For this review, take the finished solid that the model builds, in its own axes (mm). A direction names the side the tool comes from. Coordinates: 2 decimals unless noted, no trailing zeros. Loops run counter-clockwise (first coordinate to the right, second up) from the corner with the lowest first, then second, coordinate; pieces in that order, holes last. Notation, with made-up numbers: (-29.75, 4) - (5.25, 4) arc R21 ccw to (5.25, 33) - close; hole circle Ø6 at (5, -6). An arc over 180 degrees is marked (long way). One line per item, written item: value. Start each with the question number.
1. To check wall thickness, follow line 1 (X direction, y = 3.5, z = 0); line 2 (X direction, y = 0.75, z = 0); line 3 (X direction, y = 3, z = 6). State the ranges of each line that lie inside material, in increasing order. Write a range as from..to.
2. For faces 1 (the face through (8, 5.4, -8)), 2 (the face through (4.1, 4.4, 0)), 3 (the face through (7, 1.1, 5)), list the 3-axis set-ups (+Z, -Z, +X, -X, +Y, -Y) from which the entire face can be reached by the end or side of a thin tool; tool diameter is ignored.
3. Take a section at A-A, the plane x = 0. State the section outline as (y, z) points.
4. The part is to be moulded in two halves that separate along Z. For faces 4 (the face through (-5.9, 3, 10)), 5 (the face through (0, -1, 6)), 6 (the face through (-6.19, 3.28, 7.484)), 7 (the face through (-1, 3.9, -10)), say which applies: released by +Z, released by -Z, zero draft, split by the parting line, or undercut.
5. Take a section at D-D, the plane x = -8.5. State the section outline as (y, z) points, and give its area (3 significant figures).
6. Take a section at C-C, the plane y = 1.5. Count the separate pieces of the cut face and the enclosed holes in it, and give its area (3 significant figures).
7. Take a section at B-B, the plane z = 0. State the section outline as (x, y) points, and give its area (3 significant figures).
8. Insertion check: pin 1 (4 mm diameter, centred on y = 4, z = -4.5, fed in from +X); pin 2 (12 mm diameter, centred on x = 9, z = 9.5, fed in from -Y); pin 3 (2.5 mm diameter, centred on x = -2, y = 3, fed in from +Z). Each pin has a flat end and moves straight along its axis. Give the tip position at first contact, or say it passes through.
```python
from build123d import *

# Parameters (mm, degrees)
SKETCH1_R           = 12
BOSS_EXTRUDE1_DEPTH = 5.4
CUT_EXTRUDE1_START  = -4.2
CUT_EXTRUDE1_DEPTH  = 4.2
BOSS_EXTRUDE2_DEPTH = 1
SKETCH4_R           = 2.5
SKETCH4_R_2         = 2
CUT_EXTRUDE2_DEPTH  = 11
SKETCH5_R           = 2
BOSS_EXTRUDE3_DEPTH = 2
CUT_EXTRUDE3_DEPTH  = 4.3
CUT_EXTRUDE4_DEPTH  = 1.5


with BuildPart() as part:
    # Sketch1 → Boss-Extrude1 (new body)
    with BuildSketch(Plane(origin=(0, 0, 0), x_dir=(1, 0, 0), z_dir=(0, 1, 0))):
        with Locations(Location((0, 0, 0), (0, 0, 90))):
            Circle(SKETCH1_R)
    extrude(amount=BOSS_EXTRUDE1_DEPTH)

    # Sketch2 → Cut-Extrude1 (cut)
    with BuildSketch(Plane(origin=(0, 5.4, 0), x_dir=(1, 0, 0), z_dir=(0, 1, 0)).offset(CUT_EXTRUDE1_START)):
        with BuildLine():
            Line((5, -5), (5, 5))
            Line((5, 5), (-5, 5))
            Line((-5, 5), (-5, -5))
            Line((-5, -5), (-5, -8.049401897))
            Line((-5, -8.049401897), (-5.9, -8.949401897))
            Line((-5.9, -8.949401897), (-5.9, -10.449401897))
            ThreePointArc((-5.9, -10.449401897), (0, -12), (5.9, -10.449401897))
            Line((5.9, -10.449401897), (5.9, -8.949401897))
            Line((5.9, -8.949401897), (5, -8.049401897))
            Line((5, -8.049401897), (5, -5))
        make_face()
    extrude(amount=CUT_EXTRUDE1_DEPTH, mode=Mode.SUBTRACT)

    # Sketch3 → Boss-Extrude2 (add)
    with BuildSketch(Plane(origin=(0, 5.4, 0), x_dir=(1, 0, 0), z_dir=(0, 1, 0))):
        Polygon((5, -8.049401897), (3.85, -6.899401897), (3.85, 4), (-3.85, 4), (-3.85, -6.899401897), (-5, -8.049401897), (-5, 5), (5, 5), align=None)
    extrude(amount=-BOSS_EXTRUDE2_DEPTH)

    # Sketch4 → Cut-Extrude2 (cut)
    with BuildSketch(Plane(origin=(0, 5.4, 0), x_dir=(1, 0, 0), z_dir=(0, 1, 0))):
        with Locations(Location((-8, 0, 0), (0, 0, 270))):
            Circle(SKETCH4_R)
        with Locations(Location((8, 0, 0), (0, 0, 270))):
            Circle(SKETCH4_R)
        with Locations(Location((0, 8, 0), (0, 0, 270))):
            Circle(SKETCH4_R_2)
    extrude(amount=-CUT_EXTRUDE2_DEPTH, mode=Mode.SUBTRACT)

    # Sketch5 → Boss-Extrude3 (add)
    with BuildSketch(Plane.XZ):
        with Locations(Location((0, 8, 0), (0, 0, 90))):
            Circle(SKETCH5_R)
    extrude(amount=BOSS_EXTRUDE3_DEPTH)

    # Sketch6 → Cut-Extrude3 (cut)
    with BuildSketch(Plane(origin=(0, 5.4, 0), x_dir=(1, 0, 0), z_dir=(0, 1, 0))):
        with BuildLine():
            ThreePointArc((-10.796875, -2.104160221), (-9.487597374, -5.566461719), (-7.103967779, -8.398430913))
            Line((-7.103967779, -8.398430913), (-5.25, -6.544463134))
            Line((-5.25, -6.544463134), (-5.25, -2.165063509))
            ThreePointArc((-5.25, -2.165063509), (-8.038426801, -3.499789048), (-10.796875, -2.104160221))
        make_face()
        with BuildLine():
            ThreePointArc((-10.796875, 2.104160221), (-8.038426801, 3.499789048), (-5.25, 2.165063509))
            Line((-5.25, 2.165063509), (-5.25, 6))
            Line((-5.25, 6), (-2.368543856, 6))
            ThreePointArc((-2.368543856, 6), (-2.974984046, 8.871475717), (-0.915039062, 10.961875))
            ThreePointArc((-0.915039062, 10.961875), (-7.34213937, 8.191031039), (-10.796875, 2.104160221))
        make_face()
        with BuildLine():
            Line((5.25, -6.571554413), (7.089279147, -8.41083356))
            ThreePointArc((7.089279147, -8.41083356), (9.482729549, -5.574750246), (10.796875, -2.104160221))
            ThreePointArc((10.796875, -2.104160221), (8.038426801, -3.499789048), (5.25, -2.165063509))
            Line((5.25, -2.165063509), (5.25, -6.571554413))
        make_face()
        with BuildLine():
            ThreePointArc((0.915039062, 10.961875), (2.974984046, 8.871475717), (2.368543856, 6))
            Line((2.368543856, 6), (5.25, 6))
            Line((5.25, 6), (5.25, 2.165063509))
            ThreePointArc((5.25, 2.165063509), (8.038426801, 3.499789048), (10.796875, 2.104160221))
            ThreePointArc((10.796875, 2.104160221), (7.34213937, 8.191031039), (0.915039062, 10.961875))
        make_face()
    extrude(amount=-CUT_EXTRUDE3_DEPTH, mode=Mode.SUBTRACT)

    # Sketch7 → Cut-Extrude4 (cut)
    with BuildSketch(Plane(origin=(0, 5.4, 0), x_dir=(1, 0, 0), z_dir=(0, 1, 0))):
        Polygon((11.5, 2.020725942), (12.766112926, 1.289735303), (12.766112926, -1.289735303), (11.5, -2.020725942), (8, -4.041451884), (4.5, -2.020725942), (4.5, 2.020725942), (8, 4.041451884), align=None)
        Polygon((2.020725942, 4.5), (4.041451884, 8), (2.020725942, 11.5), (1.300085439, 12.748185966), (-1.300085439, 12.748185966), (-2.020725942, 11.5), (-4.041451884, 8), (-2.020725942, 4.5), align=None)
        Polygon((-4.5, -2.020725942), (-4.5, 2.020725942), (-8, 4.041451884), (-11.5, 2.020725942), (-12.378564681, 1.513486387), (-12.378564681, -1.513486387), (-11.5, -2.020725942), (-8, -4.041451884), align=None)
    extrude(amount=-CUT_EXTRUDE4_DEPTH, mode=Mode.SUBTRACT)


solid = part.part
```
Solutions:
1. line 1: -12..-10.5, -5.5..-5, 5..5.5, 10.5..12
1. line 2: -12..-10.5, -5.5..5.5, 10.5..12
1. line 3: -10.39..-9.22, -5.25..-5, 5..5.25, 9.22..10.39
2. face 1: +Z, -Z, +X, -X, +Y
2. face 2: +Z
2. face 3: +Y
3. outline: (-2, 6) - (0, 6) - (0, -6) - (3.9, -6) - (3.9, -5) - (1.2, -5) - (1.2, 12) - (0, 12) - (0, 10) - (-2, 10) - close; (0, -12) - (3.9, -12) - (3.9, -10) - (0, -10) - close; (4.4, -4.5) - (5.4, -4.5) - (5.4, -4) - (4.4, -4) - close
4. face 4: zero draft
4. face 5: split by the parting line
4. face 6: undercut
4. face 7: undercut
5. outline: (0, -8.47) - (5.4, -8.47) - (5.4, -6.98) - (1.1, -6.98) - (1.1, -3.46) - (3.9, -3.46) - (3.9, -2.45) - (0, -2.45) - close; (0, 2.45) - (3.9, 2.45) - (3.9, 3.46) - (1.1, 3.46) - (1.1, 6.98) - (5.4, 6.98) - (5.4, 8.47) - (0, 8.47) - close
5. area: 31.7 mm2
6. separate pieces: 1
6. enclosed holes: 7
6. area: 126 mm2
7. outline: (-12, 0) - (-10.5, 0) - (-10.5, 3.9) - (-12, 3.9) - close; (-5.5, 0) - (5.5, 0) - (5.5, 3.9) - (5, 3.9) - (5, 1.2) - (-5, 1.2) - (-5, 3.9) - (-5.5, 3.9) - close; (-4.5, 4.4) - (-3.85, 4.4) - (-3.85, 5.4) - (-4.5, 5.4) - close; (3.85, 4.4) - (4.5, 4.4) - (4.5, 5.4) - (3.85, 5.4) - close; (10.5, 0) - (12, 0) - (12, 3.9) - (10.5, 3.9) - close
7. area: 28.9 mm2
8. pin 1: x = 11.74
8. pin 2: y = 0
8. pin 3: z = -5
